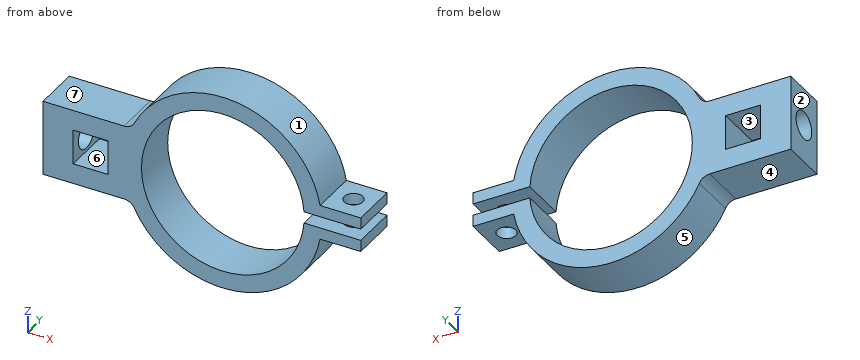
```python
from build123d import *

# Parameters (mm, degrees)
SKETCH1_W           = 7.62
SKETCH1_H           = 7.62
BOSS_EXTRUDE3_DEPTH = 10.16
CUT_EXTRUDE1_REACH  = 49.877
SKETCH5_R           = 2.032
SKETCH6_R           = 3.048
CUT_EXTRUDE2_DEPTH  = 6.604
FILLET1_R           = 2.54


with BuildPart() as part:
    # Sketch1 → Boss-Extrude3 (new body)
    with BuildSketch(Plane(origin=(0, 0, 0), x_dir=(1, 0, 0), z_dir=(0, 1, 0))):
        with BuildLine():
            Line((30.141230573, 3.809632415), (30.141230573, 1.278686529))
            Line((30.141230573, 1.278686529), (17.731545846, 1.278686529))
            ThreePointArc((17.731545846, 1.278686529), (-17.777589304, -0.008709978), (17.732790297, -1.261311079))
            Line((17.732790297, -1.261311079), (30.144338077, -1.261311079))
            Line((30.144338077, -1.261311079), (30.144338077, -3.792256965))
            Line((30.144338077, -3.792256965), (21.254338077, -3.792256965))
            ThreePointArc((21.254338077, -3.792256965), (2.324792651, -21.464469225), (-19.949513152, -8.255))
            Line((-19.949513152, -8.255), (-39.292036048, -8.255))
            Line((-39.292036048, -8.255), (-39.292036048, 8.255))
            Line((-39.292036048, 8.255), (-19.949513152, 8.255))
            ThreePointArc((-19.949513152, 8.255), (2.3160182, 21.465417762), (21.251230573, 3.809632415))
            Line((21.251230573, 3.809632415), (30.141230573, 3.809632415))
        make_face()
        with Locations((-28.878036048, -0.000367585)):
            Rectangle(SKETCH1_W, SKETCH1_H, mode=Mode.SUBTRACT)
    extrude(amount=BOSS_EXTRUDE3_DEPTH)

    # Cut-Extrude1: up to this face of the body (flat: up to its plane)
    cut_extrude1_end = Plane(part.part.faces().sort_by_distance((25.699338077, 5.08, 3.792256965))[0])
    # Sketch5 → Cut-Extrude1 (cut, up to the picked face)
    with BuildSketch(Plane(origin=(0, 0, -3.809632415), x_dir=(-1, 0, 0), z_dir=(0, 0, -1)), mode=Mode.PRIVATE) as cut_extrude1_sk1:
        with Locations((-25.696230573, 5.08)):
            Circle(SKETCH5_R)
    cut_extrude1_tool1 = split(extrude(cut_extrude1_sk1.sketch, amount=-CUT_EXTRUDE1_REACH, mode=Mode.PRIVATE), bisect_by=cut_extrude1_end, keep=Keep.BOTH, mode=Mode.PRIVATE)
    add(cut_extrude1_tool1.solids().sort_by(Axis((25.696231, 5.08, -3.809632), (0, 0, 1)))[0], mode=Mode.SUBTRACT)

    # Sketch6 → Cut-Extrude2 (cut)
    with BuildSketch(Plane.ZY.offset(39.292036048)):
        with Locations((0, 5.08)):
            Circle(SKETCH6_R)
    extrude(amount=-CUT_EXTRUDE2_DEPTH, mode=Mode.SUBTRACT)

    # Fillet1
    fillet1_edges = [part.edges().sort_by_distance(p)[0] for p in [
        (-19.949513152, 5.08, -8.255),
        (-19.949513152, 5.08, 8.255),
    ]]
    fillet(fillet1_edges, radius=FILLET1_R)


solid = part.part
```
The model under review builds one solid part; all positions refer to its coordinate system, in mm. Face numbers are marked on the shaded views. A direction names the side the tool comes from. Coordinates: 2 decimals unless noted, no trailing zeros. Write each loop counter-clockwise with the first axis right and the second up, starting at its lowest first coordinate (ties: lowest second). Pieces come first, ordered by that corner, then holes. Notation, with made-up numbers: (70.25, 62) - (87.25, 62) arc R22 cw to (87.25, 88) - close; hole circle Ø3 at (41.5, 2). An arc over 180 degrees is marked (long way). Answer in a Markdown table with one row per item. Add a question column.
Q1. To check wall thickness, follow line 1 along Z through (x, y) = (0, 6); line 2 along Z through (x, y) = (-31.5, 2) (3 decimals); line 3 along Y through (x, z) = (-37, 0). State the ranges of each line that lie inside material, in increasing order. Write a range as from..to.
Q2. Consider section B-B on y = 5.08. Give the number of separate pieces and of enclosed holes in the cut face, then the cut area to 3 significant figures.
Q3. Draft analysis for pull direction X (two halves, no side actions). For the marked faces 1, 2, 3 and 4, state which applies: +X half, -X half, draft (parallel to the pull), parting line (faces both ways), or undercut.
Q4. Consider section A-A on z = 0. Give the boundary of the cut face in (x, y).
Q5. Clearance check with flat-ended pins moving along their axes: pin 1 (5 mm diameter, centred on x = 22, y = 7, fed in from +Z); pin 2 (2 mm diameter, centred on y = 8, z = 12, fed in from -X); pin 3 (5 mm diameter, centred on x = -33.5, y = 7.5, fed in from -Z) (3 decimals); pin 4 (5 mm diameter, centred on y = 7.5, z = 5, fed in from +X). State where each tip first meets the part, or that it passes through.
Q6. For the marked faces 5, 6 and 7, list the 3-axis set-ups (+Z, -Z, +X, -X, +Y, -Y) from which the entire face can be reached by the end or side of a thin tool; tool diameter is ignored.
Q7. Consider section D-D on z = 12.5. Give the boundary of the cut face in (x, y).
Q8. Consider section C-C on x = 0. Give the boundary of the cut face in (y, z), then the cut area to 3 significant figures.
Answers below:
| question | item | result |
|---|---|---|
| 1 | line 1 | -21.59..-17.78, 17.78..21.59 |
| 1 | line 2 | -8.255..-3.81, 3.81..8.255 |
| 1 | line 3 | 0..2.03, 8.13..10.16 |
| 2 | separate pieces | 3 |
| 2 | enclosed holes | 0 |
| 2 | area | 689 mm² |
| 3 | face 1 | parting line |
| 3 | face 2 | -X half |
| 3 | face 3 | undercut |
| 3 | face 4 | draft |
| 4 | outline | (-39.29, 0) - (-32.69, 0) - (-32.69, 2.03) - (-39.29, 2.03) - close; (-39.29, 8.13) - (-32.69, 8.13) - (-32.69, 10.16) - (-39.29, 10.16) - close; (-25.07, 0) - (-17.78, 0) - (-17.78, 10.16) - (-25.07, 10.16) - close |
| 5 | pin 1 | z = 9.27 |
| 5 | pin 2 | x = -18.58 |
| 5 | pin 3 | z = -8.255 |
| 5 | pin 4 | x = 30.14 |
| 6 | face 5 | -Z, +Y, -Y |
| 6 | face 6 | +Y, -Y |
| 6 | face 7 | +Z, -X, +Y, -Y |
| 7 | outline | (-17.6, 0) - (-12.64, 0) - (-12.64, 10.16) - (-17.6, 10.16) - close; (12.64, 0) - (17.6, 0) - (17.6, 10.16) - (12.64, 10.16) - close |
| 8 | outline | (0, -21.59) - (10.16, -21.59) - (10.16, -17.78) - (0, -17.78) - close; (0, 17.78) - (10.16, 17.78) - (10.16, 21.59) - (0, 21.59) - close |
| 8 | area | 77.5 mm² |
